Here's the drawing with two shaded views (mm, measured from the low corner). I have some questions. Round coordinates to 2 decimals unless told otherwise and drop trailing zeros. Loops run counter-clockwise (first coordinate to the right, second up) from the corner with the lowest first, then second, coordinate; pieces in that order, holes last. Notation, with made-up numbers: (23.25, 63.5) -> (60.25, 63.5) arc R15 ccw to (60.25, 82.5) -> close; hole circle Ø11 at (16, 27). An arc over 180 degrees is marked (long way). Write item = value, one per line.
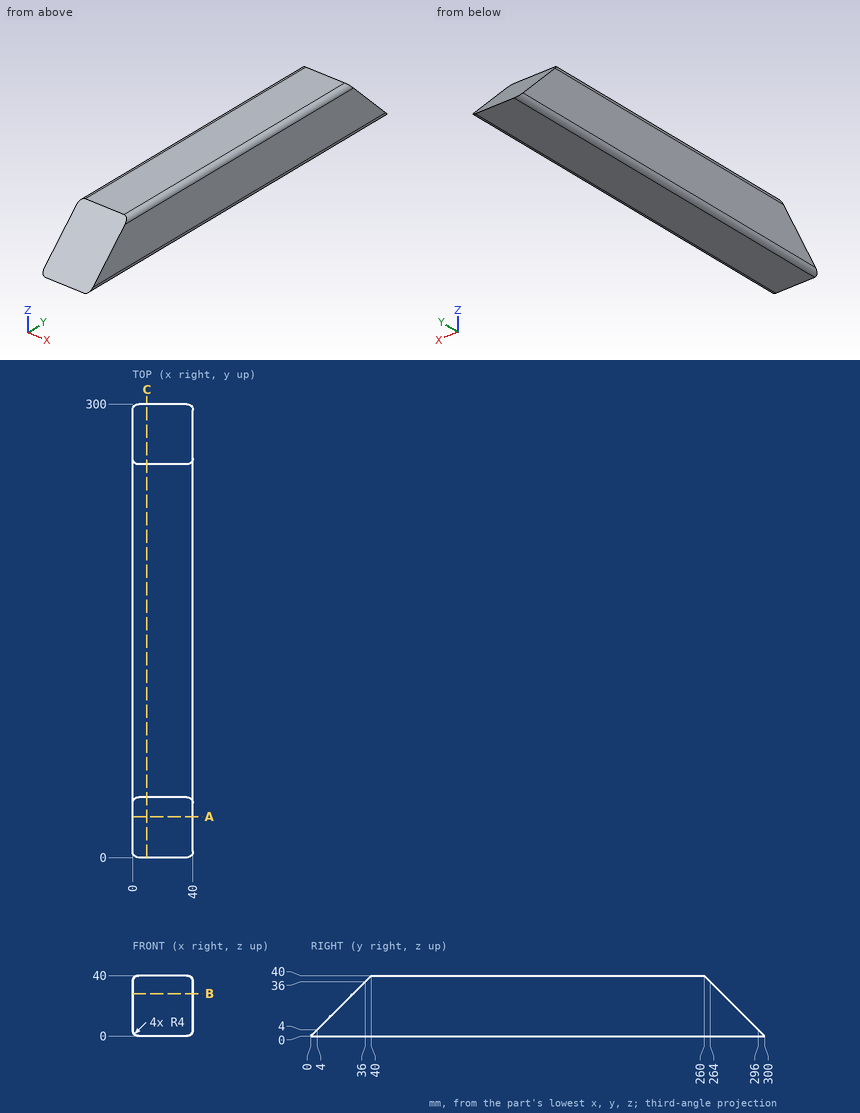
1. I'm going to push flat-ended pins straight in: pin 1 (4 mm diameter, centred on x = 23, z = 32.5, fed in from +Y); pin 2 (1.5 mm diameter, centred on x = 16.5, z = 16, fed in from -Y); pin 3 (1 mm diameter, centred on x = 18, z = 26, fed in from -Y). Where does each tip first touch, or does it pass through?
Entries:
pin_1 = 269.5
pin_2 = 15.25
pin_3 = 25.5
2. Suppose I cut it at B-B, the plane z = 28. List the corners of the cut face in (x, y) for me, and give its area (3 significant figures).
Entries:
outline = (0, 28) -> (40, 28) -> (40, 272) -> (0, 272) -> close
area = 9,760 mm²
3. Suppose I cut it at C-C, the plane x = 9.5. List the corners of the cut face in (y, z) for me, and give its area (3 significant figures).
Entries:
outline = (0, 0) -> (300, 0) -> (260, 40) -> (40, 40) -> close
area = 10,400 mm²
4. Suppose I cut it at A-A, the plane y = 27. List the corners of the cut face in (x, z) for me.
Entries:
outline = (0, 4) arc R4 ccw to (4, 0) -> (36, 0) arc R4 ccw to (40, 4) -> (40, 27) -> (0, 27) -> close
5. I need wall thicknesses on line 1 (Y direction, x = 13.5, z = 11); line 2 (Y direction, x = 2.5, z = 15.5); line 3 (Z direction, x = 20.5, y = 33). Which ranges of each line are inside material? Lowest first, please. Write a range as [from, to].
Entries:
line_1 = [11, 289]
line_2 = [15.5, 284.5]
line_3 = [0, 33]
